from build123d import *

# Parameters (mm, degrees)
SKETCH2_W           = 27
SKETCH2_H           = 49
SKETCH2_R           = 2.05
BOSS_EXTRUDE1_DEPTH = 3
SKETCH8_R           = 4.5
BOSS_EXTRUDE3_DEPTH = 3
SKETCH9_W           = 11
SKETCH9_H           = 6
CUT_EXTRUDE4_DEPTH  = 4


with BuildPart() as part:
    # Sketch2 → Boss-Extrude1 (new body)
    with BuildSketch(Plane.XY):
        with Locations((13.5, 24.5)):
            Rectangle(SKETCH2_W, SKETCH2_H)
        with Locations((6, 39)):
            Circle(SKETCH2_R, mode=Mode.SUBTRACT)
        with Locations((21, 39)):
            Circle(SKETCH2_R, mode=Mode.SUBTRACT)
        with Locations((6, 10)):
            Circle(SKETCH2_R, mode=Mode.SUBTRACT)
        with Locations((21, 10)):
            Circle(SKETCH2_R, mode=Mode.SUBTRACT)
    extrude(amount=BOSS_EXTRUDE1_DEPTH)

    # Sketch8 → Boss-Extrude3 (add)
    with BuildSketch(Plane.XY.offset(3)):
        Polygon((29.35, 0), (59.35, 0), (59.35, 49), (29.35, 49), (29.35, 46), (27, 46), (27, 26), (29.35, 26), (29.35, 23), (27, 23), (27, 3), (29.35, 3), align=None)
        with Locations((44.35, 39)):
            Circle(SKETCH8_R, mode=Mode.SUBTRACT)
        with Locations((44.35, 10)):
            Circle(SKETCH8_R, mode=Mode.SUBTRACT)
    extrude(amount=-BOSS_EXTRUDE3_DEPTH)

    # Sketch9 → Cut-Extrude4 (cut, through all)
    with BuildSketch(Plane.XY.offset(3)):
        with Locations((5.5, 24.5)):
            Rectangle(SKETCH9_W, SKETCH9_H)
        with Locations((53.85, 24.5)):
            Rectangle(SKETCH9_W, SKETCH9_H)
    extrude(amount=-CUT_EXTRUDE4_DEPTH, mode=Mode.SUBTRACT)


solid = part.part
Check sheet for the modelled part. Datum: model origin and axes. Units: mm. A direction names the side the tool comes from. Round coordinates to 2 decimals unless told otherwise and drop trailing zeros. Order: outer loops, then holes, each group sorted by start corner. A loop starts at its lowest first (then second) coordinate and runs counter-clockwise, first axis right, second up. Notation, with made-up numbers: M 7,36 L 55,36 A31 cw 55,73 Z; hole C 5,69 d2. An arc over 180 degrees is marked long. One line per item, written item: value. Start each with the question number.
1. Access from +Z, -Z, +X, -X, +Y, -Y to the whole of each face (thin tool, end or side, straight path). Record for faces 5 (the flat face through (29.35, 25, 2)), 6 (the flat face through (27, 1, 1)), 7 (the flat face through (11, 24, 2)), 8 (the flat face through (48.35, 24, 2)), 9 (the flat face through (27, 47, 1)).
2. Gauge pin test, flat ends, axial feed: P1, Ø0.9, axis at x = 5.5, z = 1.5, coming from the -Y side; P2, Ø0.9, axis at y = 23.5, z = 2, coming from the -X side; P3, Ø3.5, axis at x = 21, y = 39, coming from the +Z side; P4, Ø0.7, axis at x = 28, z = 1.5, coming from the -Y side. Record the tip position at first contact, or that the pin passes through.
3. Section check C-C on z = 0.8. Give the number of separate pieces and of enclosed holes in the cut face, and give its area (3 significant figures).
4. Scan lines: line 1 along Y through (x, z) = (21, 1.65); line 2 along Y through (x, z) = (6, 1.8); line 3 along Y through (x, z) = (44.35, 1.3). Record each from-to range of solid material in increasing order.
5. Section check D-D on x = 44.35. Enter the section's corners in (y, z), and give its area (3 significant figures).
6. Release check for a two-part mould opening along Y. For faces 1 (the flat face through (5, 27.5, 2)), 2 (the cylindrical face through (5.733, 41.033, 1.479)), 3 (the flat face through (0, 11, 1)), 4 (the flat face through (28, 46, 2)) record: released by +Y, released by -Y, zero draft, split by the parting line, or undercut.
7. Section check A-A on y = 39. Enter the section's corners in (x, z).
8. Section check B-B on x = 6. Enter the section's corners in (y, z).
Results found:
1. face 5: +Z, -Z
1. face 6: +Z, -Z, -Y
1. face 7: +Z, -Z, -X
1. face 8: +Z, -Z, +X
1. face 9: +Z, -Z, +Y
2. P1: y = 0
2. P2: x = 11
2. P3: through
2. P4: y = 3
3. separate pieces: 1
3. enclosed holes: 7
3. area: 2,570 mm^2
4. line 1: 0 to 7.95, 12.05 to 36.95, 41.05 to 49
4. line 2: 0 to 7.95, 12.05 to 21.5, 27.5 to 36.95, 41.05 to 49
4. line 3: 0 to 5.5, 14.5 to 34.5, 43.5 to 49
5. outline: M 0,0 L 5.5,0 L 5.5,3 L 0,3 Z; M 14.5,0 L 34.5,0 L 34.5,3 L 14.5,3 Z; M 43.5,0 L 49,0 L 49,3 L 43.5,3 Z
5. area: 93.0 mm^2
6. face 1: undercut
6. face 2: undercut
6. face 3: zero draft
6. face 4: released by +Y
7. outline: M 0,0 L 3.95,0 L 3.95,3 L 0,3 Z; M 8.05,0 L 18.95,0 L 18.95,3 L 8.05,3 Z; M 23.05,0 L 39.85,0 L 39.85,3 L 23.05,3 Z; M 48.85,0 L 59.35,0 L 59.35,3 L 48.85,3 Z
8. outline: M 0,0 L 7.95,0 L 7.95,3 L 0,3 Z; M 12.05,0 L 21.5,0 L 21.5,3 L 12.05,3 Z; M 27.5,0 L 36.95,0 L 36.95,3 L 27.5,3 Z; M 41.05,0 L 49,0 L 49,3 L 41.05,3 Z
